Geometry check sheet. Reference: drawing and pictorial views, mm from the part's lowest x, y, z. Round coordinates to 2 decimals unless told otherwise and drop trailing zeros. Write each loop counter-clockwise with the first axis right and the second up, starting at its lowest first coordinate (ties: lowest second). Pieces come first, ordered by that corner, then holes.
Item 1: Section check D-D, the plane x = 115. Record the cut outline in (y, z).
Item 2: Depth check by flat-ended pin: pin 1 (5 mm diameter, centred on x = 189, z = 23, fed in from +Y); pin 2 (6 mm diameter, centred on x = 161.5, y = 9.5, fed in from -Z); pin 3 (2.5 mm diameter, centred on x = 15, y = 12, fed in from +Z). Enter the tip coordinate at first touch or a pass-through.
Item 3: Material ranges on line 1 along Z through (x, y) = (225, 1.9); line 2 along Z through (x, y) = (186, 1.75); line 3 along X through (y, z) = (4.45, 77.5), recorded low to high.
Item 4: Section check A-A, the plane z = 77.5. Record the cut outline in (x, y), plus the area to 3 significant figures.
Item 5: Section check B-B, the plane y = 12. Record the cut outline in (x, z), plus the area to 3 significant figures.
Item 6: Section check C-C, the plane x = 175.5. Record the cut outline in (y, z), plus the area to 3 significant figures.
Item 7: Release check for a two-part mould opening along Z. For the marked faces 1 and 2 record: pulls with the +Z half, pulls with the -Z half, needs draft (parallel to the pull), parting line crosses it, or undercut.
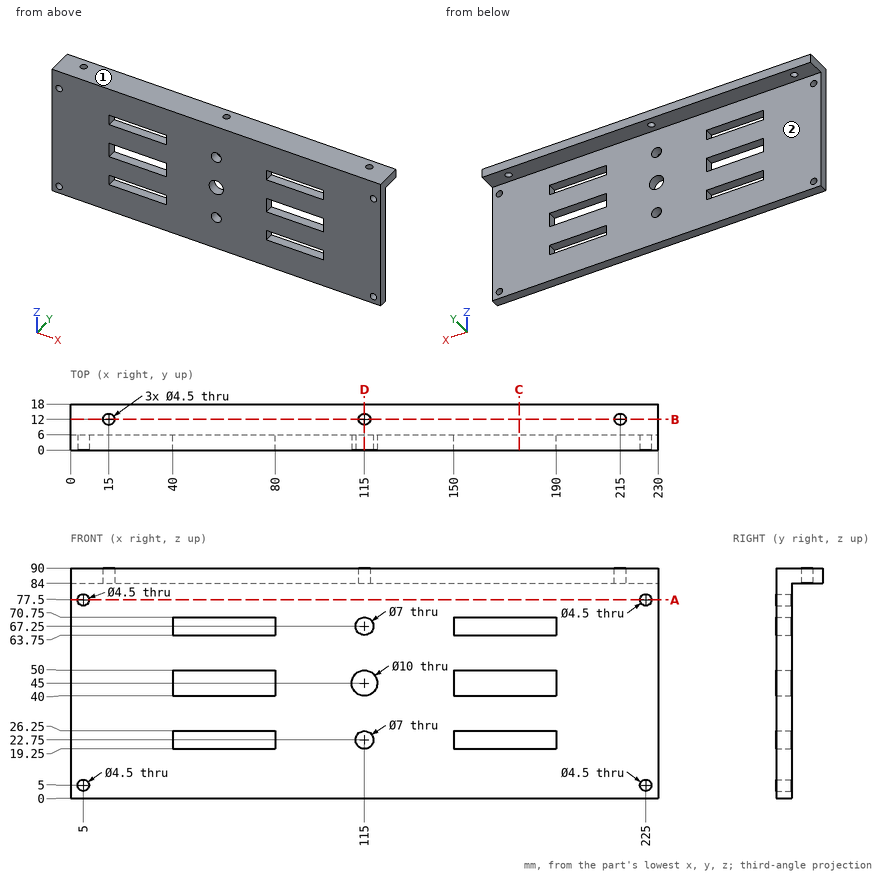
Values found:
1. outline: (0, 0) - (6, 0) - (6, 19.25) - (0, 19.25) - close; (0, 26.25) - (6, 26.25) - (6, 40) - (0, 40) - close; (0, 50) - (6, 50) - (6, 63.75) - (0, 63.75) - close; (0, 70.75) - (6, 70.75) - (6, 84) - (9.75, 84) - (9.75, 90) - (0, 90) - close; (14.25, 84) - (18, 84) - (18, 90) - (14.25, 90) - close
2. pin 1: stops at y = 6
2. pin 2: stops at z = 84
2. pin 3: passes through
3. line 1: z = 0 to 2.75, 7.25 to 75.25, 79.75 to 90
3. line 2: z = 0 to 19.25, 26.25 to 40, 50 to 63.75, 70.75 to 90
3. line 3: x = 0 to 2.75, 7.25 to 222.75, 227.25 to 230
4. outline: (0, 0) - (2.75, 0) - (2.75, 6) - (0, 6) - close; (7.25, 0) - (222.75, 0) - (222.75, 6) - (7.25, 6) - close; (227.25, 0) - (230, 0) - (230, 6) - (227.25, 6) - close
4. area: 1,330 mm2
5. outline: (0, 84) - (12.75, 84) - (12.75, 90) - (0, 90) - close; (17.25, 84) - (112.75, 84) - (112.75, 90) - (17.25, 90) - close; (117.25, 84) - (212.75, 84) - (212.75, 90) - (117.25, 90) - close; (217.25, 84) - (230, 84) - (230, 90) - (217.25, 90) - close
5. area: 1,300 mm2
6. outline: (0, 0) - (6, 0) - (6, 19.25) - (0, 19.25) - close; (0, 26.25) - (6, 26.25) - (6, 40) - (0, 40) - close; (0, 50) - (6, 50) - (6, 63.75) - (0, 63.75) - close; (0, 70.75) - (6, 70.75) - (6, 84) - (18, 84) - (18, 90) - (0, 90) - close
6. area: 468 mm2
7. face 1: pulls with the +Z half
7. face 2: needs draft
